from build123d import *

# Parameters (mm, degrees)
SKETCH_W        = 30
SKETCH_H        = 30
PAD_DEPTH       = 30
POCKET_DEPTH    = 30.001
SKETCH002_R     = 4
POCKET001_DEPTH = 30.001


with BuildPart() as part:
    # Sketch → Pad (new body)
    with BuildSketch(Plane.XZ):
        with Locations((15, 15)):
            Rectangle(SKETCH_W, SKETCH_H)
    extrude(amount=PAD_DEPTH)

    # Sketch001 (on Face3 of Pad) → Pocket (cut, through all)
    with BuildSketch(Plane(origin=(0, 0, 30), x_dir=(-1, 0, 0), z_dir=(0, 0, 1))):
        Polygon((0, 0), (0, 30), (-30, 0), align=None)
    extrude(amount=-POCKET_DEPTH, mode=Mode.SUBTRACT)

    # Sketch002 (on Face3 of Pocket) → Pocket001 (cut, through all)
    with BuildSketch(Plane(origin=(30, 0, 0), x_dir=(0, 0, 1), z_dir=(1, 0, 0))):
        with Locations((15, 15)):
            Circle(SKETCH002_R)
    extrude(amount=-POCKET001_DEPTH, mode=Mode.SUBTRACT)


solid = part.part
Geometry: final body of the model. Coordinates: model frame, mm. Give positions to 0.01 mm unless a question says otherwise; leave off trailing zeros. Write each loop counter-clockwise with the first axis right and the second up, starting at its lowest first coordinate (ties: lowest second). Pieces come first, ordered by that corner, then holes. Notation, with made-up numbers: (47.5, 6) - (96.5, 6) arc R18 cw to (96.5, 26) - close; hole circle Ø1 at (43.25, 56). An arc over 180 degrees is marked (long way). Return JSON: item names as keys, results as strings. Group by question number.
1) Line query: line 1 (Z direction, x = 22.25, y = -15); line 2 (X direction, y = -19, z = 14.5); line 3 (Y direction, x = 18.5, z = 15). Output: solid intervals per line, ascending.
2) First-contact query: P1, Ø2, axis at x = 10, z = 18.5, coming from the +Y side; P2, Ø3, axis at y = -26, z = 26.5, coming from the -X side; P3, Ø6, axis at y = -7.5, z = 3, coming from the -X side. Flat tips, straight axial feed; report the tip coordinate or a pass-through.
3) Section B-B on z = 15. Return the cut outline in (x, y), plus the area to 3 significant figures.
4) Section A-A on y = -15. Return the cut outline in (x, z).
5) Section D-D on z = 4. Return the cut outline in (x, y).
6) Section C-C on x = 25. Return the cut outline in (y, z), plus the area to 3 significant figures.
7) Mould query, pull axis Z, two halves, no side actions, for faces 1 (the flat face through (21, -21, 0)), 2 (the cylindrical face through (22.744, -18.966, 14.479)), 3 (the flat face through (15, -30, 15)). Classes: released by +Z, released by -Z, zero draft, split by the parting line, or undercut.
Filled in:
{
 "1": {"line 1": "z = 0 to 11, 19 to 30", "line 2": "x = 11 to 30", "line 3": "y = -30 to -19"},
 "2": {"P1": "stops at y = -19", "P2": "stops at x = 2.5", "P3": "stops at x = 19.5"},
 "3": {"outline": "(0, -30) - (30, -30) - (30, -19) - (11, -19) - close; (19, -11) - (30, -11) - (30, 0) - close", "area": "330 mm^2"},
 "4": {"outline": "(15, 0) - (30, 0) - (30, 11) - (15, 11) - close; (15, 19) - (30, 19) - (30, 30) - (15, 30) - close"},
 "5": {"outline": "(0, -30) - (30, -30) - (30, 0) - close"},
 "6": {"outline": "(-30, 0) - (-5, 0) - (-5, 30) - (-30, 30) - close; hole circle Ø8 at (-15, 15)", "area": "700 mm^2"},
 "7": {"face 1": "released by -Z", "face 2": "undercut", "face 3": "zero draft"}
}
